from build123d import *

# Parameters (mm, degrees)
BOSS_EXTRU_1_DEPTH      = 10
ESQUISSE2_R             = 2.5
ENL_V_MAT_EXTRU_1_DEPTH = 42.821047333


with BuildPart() as part:
    # Esquisse1 → Boss.-Extru.1 (new body)
    with BuildSketch(Plane.XY):
        Polygon((0, 0), (40, 1), (40, -7), (0, -6), align=None)
    extrude(amount=BOSS_EXTRU_1_DEPTH)

    # Esquisse2 → Enlèv. mat.-Extru.1 (cut, through all)
    with BuildSketch(Plane(origin=(0, 0, 0), x_dir=(0.9996876464081228, 0.024992191160203233, 0), z_dir=(-0.02499219116020323, 0.9996876464081227, 0))):
        with Locations(Location((5, -5, 0), (0, 0, 180))):
            Circle(ESQUISSE2_R)
        with Locations(Location((35.012498047, -5, 0), (0, 0, 180))):
            Circle(ESQUISSE2_R)
    extrude(amount=-ENL_V_MAT_EXTRU_1_DEPTH, mode=Mode.SUBTRACT)


solid = part.part
The listing builds one solid part. Answer for the finished solid, in the listing's coordinates (mm). A direction names the side the tool comes from. Coordinates: 2 decimals unless noted, no trailing zeros. Write each loop counter-clockwise with the first axis right and the second up, starting at its lowest first coordinate (ties: lowest second). Pieces come first, ordered by that corner, then holes. Notation, with made-up numbers: M -12,26 L 28,26 A13 ccw 28,50 Z; hole C 18,-12 d8. An arc over 180 degrees is marked long. Put each result on its own line as item: value. Start each with the question number.
1. A cutting plane is placed at A-A on z = 6. Write down the section's boundary in (x, y).
2. A cutting plane is placed at C-C on z = 1. Write down the section's boundary in (x, y), then the cut area to 3 significant figures.
3. Consider line 1 (X direction, y = -4.25, z = 6.25); line 2 (X direction, y = -3, z = 3); line 3 (Z direction, x = 5, y = 0). Determine where each line is inside the solid, lowest interval first. Write a range as from..to.
4. Which of the six approach directions +Z, -Z, +X, -X, +Y, -Y give full straight-line access (tool end or side, diameter ignored) to faces 5 (the flat face through (20, -3, 0)), 6 (the cylindrical face through (5.4, -3.02, 7.48))?
5. A flat-ended cylindrical pin translates along its axis: P1, Ø3, axis at x = 23, z = 5, coming from the +Y side. Find the tip coordinate at first contact, or state that the pin passes through.
6. A cutting plane is placed at B-B on x = 24. Write down the section's boundary in (y, z), then the cut area to 3 significant figures.
7. A cutting plane is placed at D-D on y = -1.5. Count the separate pieces of the cut face and the enclosed holes in it, then the cut area to 3 significant figures.
8. For a pull along X with two mould halves and no side action, classify faces 1 (the cylindrical face through (37.596, -2.953, 5.11)), 2 (the flat face through (40, -3, 5)), 3 (the flat face through (0, -3, 5)), 4 (the flat face through (20, -3, 10)) as pulls with the +X half, pulls with the -X half, needs draft (parallel to the pull), parting line crosses it, or undercut.
Resolved:
1. outline: M 0,-6 L 2.86,-6.07 L 2.71,0.07 L 0,0 Z; M 7.29,0.18 L 7.45,-6.19 L 32.9,-6.82 L 32.71,0.82 Z; M 37.29,0.93 L 37.49,-6.94 L 40,-7 L 40,1 Z
2. outline: M 0,-6 L 40,-7 L 40,1 L 0,0 Z
2. area: 280 mm2
3. line 1: x = 0..2.94, 7.27..32.96, 37.3..40
3. line 2: x = 0..3.58, 6.58..33.6, 36.6..40
3. line 3: z = 0..2.5, 7.5..10
4. face 5: -Z, +X, -X, +Y, -Y
4. face 6: none
5. P1: stops at y = 0.61
6. outline: M -6.6,0 L 0.6,0 L 0.6,10 L -6.6,10 Z
6. area: 72.0 mm2
7. separate pieces: 1
7. enclosed holes: 2
7. area: 361 mm2
8. face 1: undercut
8. face 2: pulls with the +X half
8. face 3: pulls with the -X half
8. face 4: needs draft
